Input: part model. Units: mm. Frame: model coordinates. A direction names the side the tool comes from. Round coordinates to 2 decimals unless told otherwise and drop trailing zeros. Loops run counter-clockwise (first coordinate to the right, second up) from the corner with the lowest first, then second, coordinate; pieces in that order, holes last. Notation, with made-up numbers: M 55.5,79 L 107.5,79 A17 cw 107.5,99 Z; hole C 41.5,62.25 d2. An arc over 180 degrees is marked long. Use one line per item in the form item = value. Start each with the question number.
Q1. Mould query, pull axis Y, two halves, no side actions, for faces 1 (the flat face through (0, 0, 17.125)), 2 (the cylindrical face through (-1.43, -0.45, -1.55)), 3 (the flat face through (0, 2, 19)), 4 (the flat face through (0.616, -1.088, 18.076)). Classes: pulls with the +Y half, pulls with the -Y half, needs draft (parallel to the pull), parting line crosses it, or undercut.
Q2. Access query for faces 5 (the cylindrical face through (0.596, 2.685, 17.413)), 6 (the flat face through (-2, 0, 16)), 7 (the flat face through (-0.63, -1.08, 18.08)). Directions: +Z, -Z, +X, -X, +Y, -Y. A direction counts if a zero-diameter tool reaches every point of the face in a straight line with its end or side. Return the directions, or none.
Q3. First-contact query: P1, Ø1.2, axis at x = -0.5, y = -0.5, coming from the +Z side; P2, Ø1.5, axis at x = -0.5, z = -3.5, coming from the +Y side; P3, Ø3, axis at x = 1.5, z = -15, coming from the -Y side. Flat tips, straight axial feed; report the tip coordinate or a pass-through.
Q4. Section query B-B, the plane z = 1.5. Output: boundary loops of the cut face in (x, y).
Q5. Ray query, line 1 along Z through (x, y) = (-1.4, -1.85); line 2 along X through (y, z) = (-0.1, 13). Return the intervals inside material, ascending.
```python
from build123d import *

# Parameters (mm, degrees)
CUT_EXTRUDE1_DEPTH = 1.875
CHAMFER1_SIZE      = 0.275
CHAMFER2_SIZE      = 0.1375
CHAMFER3_SIZE      = 0.375


with BuildPart() as part:
    # Sketch2 → Revolve1 (revolve)
    with BuildSketch(Plane(origin=(0, 0, 0), x_dir=(0, 0, -1), z_dir=(1, 0, 0)), mode=Mode.PRIVATE) as revolve1_sk:
        Polygon((-19, 2.75), (-16, 2.75), (-16, 1.5), (19, 1.5), (19, 0), (-19, 0), align=None)
    revolve(revolve1_sk.sketch.rotate(Axis((0, 0, -19), (0, 0, 1)), 90), axis=Axis((0, 0, -19), (0, 0, 1)))

    # Sketch4 → Cut-Extrude1 (cut)
    with BuildSketch(Plane.XY.offset(19)):
        Polygon((0, 1.443375673), (-1.25, 0.721687836), (-1.25, -0.721687836), (0, -1.443375673), (1.25, -0.721687836), (1.25, 0.721687836), align=None)
    extrude(amount=-CUT_EXTRUDE1_DEPTH, mode=Mode.SUBTRACT)

    # Cut-Extrude2 cone 1 section (on through the dimple's axis) → Cut-Extrude2 (revolve, cut)
    with BuildSketch(Plane(origin=(0, 0, 19), x_dir=(0, -1, 0), z_dir=(1, 0, 0))):
        Polygon((0, 0), (1.443375673, 0), (0, 0.833333333), align=None)
    revolve(axis=Axis((0, 0, 19), (0, 0, -1)), mode=Mode.SUBTRACT)

    # Chamfer1
    chamfer1_edges = [part.edges().sort_by_distance(p)[0] for p in [
        (2.75, 0, 19),
    ]]
    chamfer(chamfer1_edges, length=CHAMFER1_SIZE)

    # Chamfer2
    chamfer2_edges = [part.edges().sort_by_distance(p)[0] for p in [
        (2.75, 0, 16),
    ]]
    chamfer(chamfer2_edges, length=CHAMFER2_SIZE)

    # Chamfer3
    chamfer3_edges = [part.edges().sort_by_distance(p)[0] for p in [
        (1.5, 0, -19),
    ]]
    chamfer(chamfer3_edges, length=CHAMFER3_SIZE)


solid = part.part
```
Results found:
q1.face_1 = undercut
q1.face_2 = parting line crosses it
q1.face_3 = needs draft
q1.face_4 = undercut
q2.face_5 = +Z, -Z
q2.face_6 = -Z
q2.face_7 = +Z
q3.P1 = 18.92
q3.P2 = 1.5
q3.P3 = -1.5
q4.outline = C 0,0 d3
q5.line_1 = 16 to 19
q5.line_2 = -1.5 to 1.5
